from build123d import *

# Parameters (mm, degrees)
CROQUIS1_R = 13.7


with BuildPart() as part:
    # Barrer1: sweep along a curve in space
    with BuildLine() as barrer1_path:
        Line((0, 0, 0), (-185, 0, 0))
        ThreePointArc((-185, 0, 0), (-195.606601718, 4.393398282, 0), (-200, 15, 0))
        Line((-200, 15, 0), (-200, 285, 0))
        ThreePointArc((-200, 300, -15), (-200, 295.606601718, -4.393398282), (-200, 285, 0))
        Line((-200, 300, -15), (-200, 300, -950))
        ThreePointArc((-200, 350, -1000), (-200, 314.644660941, -985.355339059), (-200, 300, -950))
        Line((-200, 464, -1000), (-200, 350, -1000))
        ThreePointArc((-200, 464, -1000), (-200, 499.355339059, -1014.644660941), (-200, 514, -1050))
        Line((-200, 514, -1050), (-200, 514, -1591))
        ThreePointArc((-200, 514, -1591), (-195.606601718, 514, -1601.606601718), (-185, 514, -1606))
        Line((-185, 514, -1606), (-30, 514, -1606))
    # Croquis1 → Barrer1 (sweep)
    with BuildSketch(Plane(origin=(0, 0, 0), x_dir=(0, 0, -1), z_dir=(1, 0, 0))):
        Circle(CROQUIS1_R)
    sweep(path=barrer1_path.line)


solid = part.part
Input: part model. Units: mm. Frame: model coordinates. A direction names the side the tool comes from. Give positions to 0.01 mm unless a question says otherwise; leave off trailing zeros. Write each loop counter-clockwise with the first axis right and the second up, starting at its lowest first coordinate (ties: lowest second). Pieces come first, ordered by that corner, then holes.
Q1. Set-up query: faces 4 (the face through (-106.415, 516.97, -1592.626)), 5 (the face through (0, 0, 0)), 6 (the face through (-204.115, 407.798, -1013.067)). Return all of +Z, -Z, +X, -X, +Y, -Y with unobstructed straight access to the full face (end or side cutting, diameter ignored); none if empty.
Q2. Section B-B, the plane x = -138.5. Output: boundary loops of the cut face in (y, z), plus the area to 3 significant figures.
Q3. Section A-A, the plane y = 236.5. Output: boundary loops of the cut face in (x, z).
Q4. Material intervals for probe 1 along Z at (x, y) = (-195, 53) (3 decimals), sorted ascending.
Q5. Pull-direction query (Y, two-part tool) for faces 1 (the face through (-93.795, -9.259, 10.097)), 2 (the face through (-30, 514, -1606)), 3 (the face through (-213.583, 151.89, 1.783)); classes: pulls with the +Y half, pulls with the -Y half, needs draft (parallel to the pull), parting line crosses it, or undercut.
Q6. First-contact query: P1, Ø13.5, axis at y = 519, z = -1611.5, coming from the +X side. Flat tip, straight axial feed; report the tip coordinate or a pass-through.
Filled in:
1. face 4: +X
1. face 5: +Z, -Z, +X, +Y, -Y
1. face 6: none
2. outline: circle Ø27.4 at (0, 0); circle Ø27.4 at (514, -1606)
2. area: 1,180 mm2
3. outline: circle Ø27.4 at (-200, 0)
4. probe 1: z = -12.755 to 12.755
5. face 1: parting line crosses it
5. face 2: needs draft
5. face 3: undercut
6. P1: stops at x = -30
